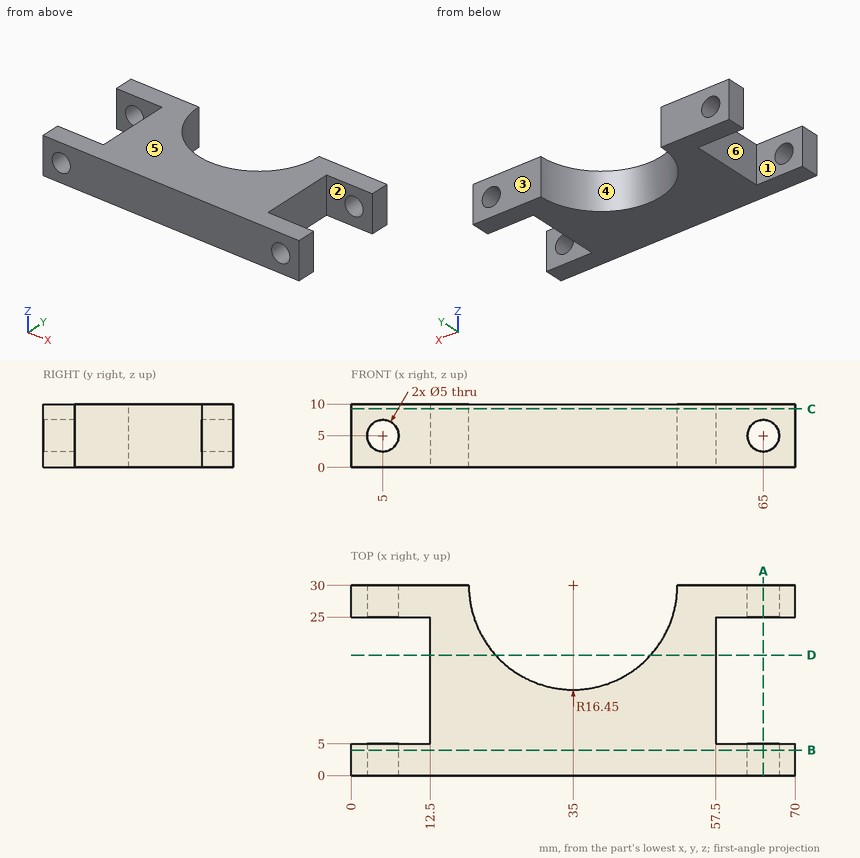
Study the drawing (mm; zero at the part's minimum x, y, z) and answer. A direction names the side the tool comes from. Give positions to 0.01 mm unless a question says otherwise; leave off trailing zeros. Loops run counter-clockwise (first coordinate to the right, second up) from the corner with the lowest first, then second, coordinate; pieces in that order, holes last. Notation, with made-up numbers: (16.25, 21) -> (45.25, 21) arc R13 ccw to (45.25, 38) -> close; hole circle Ø10 at (24.5, -33.75). An arc over 180 degrees is marked (long way). Use a Markdown table: item, result. Add a question column.
1) Consider line 1 along Z through (x, y) = (65, 26.5); line 2 along Y through (x, z) = (8, 3.25); line 3 along X through (y, z) = (11, 4.5). Determine where each line is inside the solid, lowest interval first.
2) The part is cut by section B-B, the plane y = 4. Determine the outline of the cut face in (x, z), plus the area to 3 significant figures.
3) The part is cut by section C-C, the plane z = 9.25. Determine the outline of the cut face in (x, y), plus the area to 3 significant figures.
4) Each of these flat-tipped pins is pushed along its axis until it touches: P1, Ø6, axis at x = 62.5, y = 16, coming from the +Z side; P2, Ø3, axis at y = 13.5, z = 6, coming from the -X side. Where does it stop, or does it pass through?
5) For a pull along Y with two mould halves and no side action, classify the marked faces 4, 5 and 6 as +Y half, -Y half, draft (parallel to the pull), parting line (faces both ways), or undercut.
6) The part is cut by section A-A, the plane x = 65. Determine the outline of the cut face in (y, z).
7) The part is cut by section D-D, the plane y = 19. Determine the outline of the cut face in (x, z).
8) Which of the six approach directions +Z, -Z, +X, -X, +Y, -Y give full straight-line access (tool end or side, diameter ignored) to the marked faces 1, 2 and 3?
Reported:
| question | item | result |
|---|---|---|
| 1 | line 1 | z = 0 to 2.5, 7.5 to 10 |
| 1 | line 2 | y = 0 to 5, 25 to 30 |
| 1 | line 3 | x = 12.5 to 57.5 |
| 2 | outline | (0, 0) -> (70, 0) -> (70, 10) -> (0, 10) -> close; hole circle Ø5 at (5, 5); hole circle Ø5 at (65, 5) |
| 2 | area | 661 mm^2 |
| 3 | outline | (0, 0) -> (70, 0) -> (70, 5) -> (57.5, 5) -> (57.5, 25) -> (70, 25) -> (70, 30) -> (51.45, 30) arc R16.45 cw to (18.55, 30) -> (0, 30) -> (0, 25) -> (12.5, 25) -> (12.5, 5) -> (0, 5) -> close |
| 3 | area | 1,170 mm^2 |
| 4 | P1 | passes through |
| 4 | P2 | stops at x = 12.5 |
| 5 | face 4 | +Y half |
| 5 | face 5 | draft |
| 5 | face 6 | undercut |
| 6 | outline | (0, 0) -> (5, 0) -> (5, 2.5) -> (0, 2.5) -> close; (0, 7.5) -> (5, 7.5) -> (5, 10) -> (0, 10) -> close; (25, 0) -> (30, 0) -> (30, 2.5) -> (25, 2.5) -> close; (25, 7.5) -> (30, 7.5) -> (30, 10) -> (25, 10) -> close |
| 7 | outline | (12.5, 0) -> (22.77, 0) -> (22.77, 10) -> (12.5, 10) -> close; (47.23, 0) -> (57.5, 0) -> (57.5, 10) -> (47.23, 10) -> close |
| 8 | face 1 | +Z, -Z, -X |
| 8 | face 2 | +Z, -Z, +X |
| 8 | face 3 | +Z, -Z, +X, -X, +Y |
